Design review of the part built by this model. Coordinates are the model's own, in mm. A direction names the side the tool comes from. Round coordinates to 2 decimals unless told otherwise and drop trailing zeros. Order: outer loops, then holes, each group sorted by start corner. A loop starts at its lowest first (then second) coordinate and runs counter-clockwise, first axis right, second up. Notation, with made-up numbers: (-3.5, 85) - (8.5, 85) arc R28 cw to (8.5, 108) - close; hole circle Ø2 at (53.5, 14). An arc over 180 degrees is marked (long way). Use CSV: the item, a comma, the result in double quotes.
Autodesk Inventor part; units mm, degrees
ref_plane "YZ Plane" through (0, 0, 0) normal (1, 0, 0) x (0, 1, 0)
ref_plane "XZ Plane" through (0, 0, 0) normal (0, 1, 0) x (-1, 0, 0)
ref_plane "XY Plane" through (0, 0, 0) normal (0, 0, 1) x (1, 0, 0)
sketch "Sketch1" plane through (0, 0, 0) normal (0, 0, 1) x (1, 0, 0)
  line L0 (25, -2.55) -> (-25, -2.55)
  line L1 (-25, -2.55) -> (-25, 2.55)
  line L2 (-25, 2.55) -> (25, 2.55)
  line L3 (25, 2.55) -> (25, -2.55)
  line L4 (25, -2.55) -> (-25, 2.55) construction
  line L5 (-25, -2.55) -> (25, 2.55) construction
  point P0 (0, 0)
  dimension "d0" = 50
  dimension "d1" = 5.1
extrude "Extrusion1" add sketch "Sketch1" along normal blind 45.1
sketch "Sketch2" plane through (-25, -2.55, 0) normal (0, -1, 0) x (1, 0, 0)
  line L0 (50, 0) -> (0, 0)
  line L1 (9.85, 0) -> (15.35, 0)
  line L2 (15.35, 0) -> (15.35, 5.1)
  line L3 (15.35, 5.1) -> (9.85, 5.1)
  line L4 (9.85, 5.1) -> (9.85, 0)
  line L5 (40.15, 0) -> (34.65, 0)
  line L6 (34.65, 0) -> (34.65, 5.1)
  line L7 (34.65, 5.1) -> (40.15, 5.1)
  line L8 (40.15, 5.1) -> (40.15, 0)
  line L9 (50, 0) -> (50, 45.1)
  line L10 (0, 0) -> (0, 45.1)
  point P0 (25, 0)
  point P1 (40.15, 2.55)
  dimension "d5" = 5.1
  dimension "d9" = 5.1
  dimension "d17" = 9.85
  dimension "d25" = 5.5
  dimension "d26" = 5.5
  dimension "d27" = 9.85
extrude "Extrusion2" cut sketch "Sketch2" against normal blind 45.1
sketch "Sketch3" plane through (-25, -2.55, 45.1) normal (0, -1, 0) x (1, 0, 0)
  circle A0 centre (25, -5.6) radius 3.45
  line L0 (0, 0) -> (50, 0)
  circle A1 centre (25, -5.6) radius 12.05
  line L1 (50, 0) -> (0, 0)
  line L2 (0, 0) -> (0, 10.45)
  line L3 (0, 10.45) -> (50, 10.45)
  line L4 (50, 10.45) -> (50, 0)
  line L5 (0, -45.1) -> (0, 0)
  point P0 (25, -45.1)
  point P1 (14.3303, 0)
  point P2 (35.6697, 0)
  dimension "d12" = 6.9
  dimension "d13" = 5.6
  dimension "d14" = 25
  dimension "d19" = 24.1
  dimension "d20" = 16.05
extrude "Extrusion3" cut sketch "Sketch3" against normal blind 45.1 contours A0 | L0 A1 picked at (25.1386, -0.7251)
extrude "Extrusion4" add sketch "Sketch3" against normal up to surface (5.1 mm away) contours L2 L3 L4 L0 A1
fillet "Fillet1" radius 15 2 edges at (25, 0, 55.55) (-25, 0, 55.55)
equation "\"d26\" = d25"
equation "\"d27\" = d17"
properties part number "motorholder1A" material "Polycarbonate, Smoke"
1) We need section B-B (x = 0). Give the boundary of the cut face in (y, z), then the cut area to 3 significant figures.
Data:
outline,"(-2.55, 0) - (2.55, 0) - (2.55, 27.45) - (-2.55, 27.45) - close; (-2.55, 51.55) - (2.55, 51.55) - (2.55, 55.55) - (-2.55, 55.55) - close"
area,"160 mm2"
2) The part is to be moulded in two halves that separate along X. For faces 3 (the face through (0, 0, 0)), 4 (the face through (-12, 0, 5.1)), 5 (the face through (-25, 0, 20)), say which applies: +X half, -X half, draft (parallel to the pull), parting line (faces both ways), or undercut.
Data:
face 3,"draft"
face 4,"undercut"
face 5,"-X half"
3) We need section D-D (x = -20). Give the boundary of the cut face in (y, z), then the cut area to 3 significant figures.
Data:
outline,"(-2.55, 0) - (2.55, 0) - (2.55, 51.73) - (-2.55, 51.73) - close"
area,"264 mm2"
4) For faces 1 (the face through (-9.65, 0, 3)), 2 (the face through (-20, 0, 0)), list the 3-axis set-ups (+Z, -Z, +X, -X, +Y, -Y) from which the entire face can be reached by the end or side of a thin tool; tool diameter is ignored.
Data:
face 1,"-Z, +Y, -Y"
face 2,"-Z, +X, -X, +Y, -Y"
5) To check wall thickness, follow L1, parallel to X at y = 1.4, z = 39.5; L2, parallel to Z at x = 0, y = 0.75; L3, parallel to Z at x = -9, y = -0.6. State the ranges of each line that lie inside material, in increasing order. Write a range as from..to.
Data:
L1,"x = -25..-12.05, 12.05..25"
L2,"z = 0..27.45, 51.55..55.55"
L3,"z = 0..31.49, 47.51..55.55"
6) We need section A-A (z = 39.5). Give the boundary of the cut face in (x, y), then the cut area to 3 significant figures.
Data:
outline,"(-25, -2.55) - (-12.05, -2.55) - (-12.05, 2.55) - (-25, 2.55) - close; (12.05, -2.55) - (25, -2.55) - (25, 2.55) - (12.05, 2.55) - close"
area,"132 mm2"
7) We need section C-C (y = -1.45). Give the boundary of the cut face in (x, z).
Data:
outline,"(-25, 0) - (-15.15, 0) - (-15.15, 5.1) - (-9.65, 5.1) - (-9.65, 0) - (9.65, 0) - (9.65, 5.1) - (15.15, 5.1) - (15.15, 0) - (25, 0) - (25, 40.55) arc R15 ccw to (10, 55.55) - (-10, 55.55) arc R15 ccw to (-25, 40.55) - close; hole circle Ø24.1 at (0, 39.5)"
8) Insertion check: pin 1 Ø19.5 at (x, z) = (0, 39.5) entering from -Y; pin 2 Ø1.5 at (x, y) = (12, 0.5) entering from -Z. Each pin has a flat end and moves straight along its axis. Give the tip position at first contact, or say it passes through.
Data:
pin 1,"passes through"
pin 2,"stops at z = 5.1"
